The model under review builds one solid part; all positions refer to its coordinate system, in mm. A direction names the side the tool comes from. Coordinates: 2 decimals unless noted, no trailing zeros. Order: outer loops, then holes, each group sorted by start corner. A loop starts at its lowest first (then second) coordinate and runs counter-clockwise, first axis right, second up. Notation, with made-up numbers: (17.25, 17.5) -> (72.25, 17.5) arc R14 cw to (72.25, 31.5) -> close; hole circle Ø11 at (84, 83.5). An arc over 180 degrees is marked (long way). Use one line per item in the form item = value. Start each with the question number.
(1) Mouldability with a two-part tool opening along Z and no side actions: class faces 3 (the flat face through (0, 2, -6)), 4 (the flat face through (-5.3, 5, -4.1)), 5 (the cylindrical face through (1.352, 2.606, 4.292)) as +Z half, -Z half, draft (parallel to the pull), parting line (faces both ways), or undercut.
(2) Take a section at A-A (y = 3.5). State the section outline as (x, z) points, then the cut area to 3 significant figures.
(3) Take a section at C-C (x = 7). State the section outline as (y, z) points, then the cut area to 3 significant figures.
(4) Take a section at D-D (y = 1.45). State the section outline as (x, z) points.
(5) Wall thickness on line 1 along X through (y, z) = (0.95, 0); line 2 along Z through (x, y) = (0, 2.5); line 3 along X through (y, z) = (2.75, 0): over which ranges is each line inside the solid? List them lowest first.
(6) Insertion check: pin 1 Ø4.5 at (x, z) = (-7, 1) entering from +Y. The pin has a flat end and moves straight along its axis. Give the tip position at first contact, or say it passes through.
(7) Take a section at B-B (z = 0.5). State the section outline as (x, y) points.
(8) For faces 1 (the flat face through (-22.5, 2, 0)), 2 (the cylindrical face through (-20.15, 4.01, -0.06)), list the 3-axis set-ups (+Z, -Z, +X, -X, +Y, -Y) from which the entire face can be reached by the end or side of a thin tool; tool diameter is ignored.
```python
from build123d import *

# Parameters (mm, degrees)
SKETCH1_W           = 45
SKETCH1_H           = 12
BOSS_EXTRUDE1_DEPTH = 5
SKETCH2_R           = 2.65
CUT_EXTRUDE1_DEPTH  = 2
SKETCH3_R           = 1.65
CUT_EXTRUDE2_DEPTH  = 12
SKETCH4_R           = 4.5
CUT_EXTRUDE3_DEPTH  = 0.8


with BuildPart() as part:
    # Sketch1 → Boss-Extrude1 (new body)
    with BuildSketch(Plane(origin=(0, 0, 0), x_dir=(1, 0, 0), z_dir=(0, 1, 0))):
        Rectangle(SKETCH1_W, SKETCH1_H)
    extrude(amount=BOSS_EXTRUDE1_DEPTH)

    # Sketch2 → Cut-Extrude1 (cut)
    with BuildSketch(Plane(origin=(0, 5, 0), x_dir=(1, 0, 0), z_dir=(0, 1, 0))):
        with Locations((-17.5, 0)):
            Circle(SKETCH2_R)
        with BuildLine():
            Line((-0.940913384, 4.400532014), (-17.5, 2.65))
            ThreePointArc((-17.5, 2.65), (-15.62616703, 1.87383297), (-14.85, 0))
            ThreePointArc((-14.85, 0), (-15.62616703, -1.87383297), (-17.5, -2.65))
            Line((-17.5, -2.65), (-0.940913384, -4.400532014))
            ThreePointArc((-0.940913384, -4.400532014), (-4.5, 0), (-0.940913384, 4.400532014))
        make_face()
        with BuildLine():
            Line((0, 4.5), (-0.940913384, 4.400532014))
            ThreePointArc((-0.940913384, 4.400532014), (-4.5, 0), (-0.940913384, -4.400532014))
            Line((-0.940913384, -4.400532014), (0, -4.5))
            Line((0, -4.5), (0.940913384, -4.400532014))
            ThreePointArc((0.940913384, -4.400532014), (3.498864832, -2.829831247), (4.5, 0))
            ThreePointArc((4.5, 0), (3.498864832, 2.829831247), (0.940913384, 4.400532014))
            Line((0.940913384, 4.400532014), (0, 4.5))
        make_face()
        with BuildLine():
            Line((17.5, 2.65), (0.940913384, 4.400532014))
            ThreePointArc((0.940913384, 4.400532014), (3.498864832, 2.829831247), (4.5, 0))
            ThreePointArc((4.5, 0), (3.498864832, -2.829831247), (0.940913384, -4.400532014))
            Line((0.940913384, -4.400532014), (17.5, -2.65))
            ThreePointArc((17.5, -2.65), (14.85, 0), (17.5, 2.65))
        make_face()
        with Locations((17.5, 0)):
            Circle(SKETCH2_R)
    extrude(amount=-CUT_EXTRUDE1_DEPTH, mode=Mode.SUBTRACT)

    # Sketch3 → Cut-Extrude2 (cut)
    with BuildSketch(Plane(origin=(0, 3, 0), x_dir=(1, 0, 0), z_dir=(0, 1, 0))):
        with Locations(Location((0, 0, 0), (0, 0, 270))):
            Circle(SKETCH3_R)
    extrude(amount=-CUT_EXTRUDE2_DEPTH, mode=Mode.SUBTRACT)

    # Sketch4 → Cut-Extrude3 (cut)
    with BuildSketch(Plane(origin=(0, 3, 0), x_dir=(1, 0, 0), z_dir=(0, 1, 0))):
        with Locations(Location((0, 0, 0), (0, 0, 270))):
            Circle(SKETCH4_R)
    extrude(amount=-CUT_EXTRUDE3_DEPTH, mode=Mode.SUBTRACT)


solid = part.part
```
Findings:
q1.face_3 = -Z half
q1.face_4 = draft
q1.face_5 = undercut
q2.outline = (-22.5, -6) -> (22.5, -6) -> (22.5, 6) -> (-22.5, 6) -> close; hole (-17.5, -2.65) -> (0, -4.5) -> (17.5, -2.65) arc R2.65 ccw to (17.5, 2.65) -> (0, 4.5) -> (-17.5, 2.65) arc R2.65 ccw to start
q2.area = 268 mm²
q3.outline = (0, -6) -> (5, -6) -> (5, -3.76) -> (3, -3.76) -> (3, 3.76) -> (5, 3.76) -> (5, 6) -> (0, 6) -> close
q3.area = 45.0 mm²
q4.outline = (-22.5, -6) -> (22.5, -6) -> (22.5, 6) -> (-22.5, 6) -> close; hole circle Ø3.3 at (0, 0)
q5.line_1 = -22.5 to -1.65, 1.65 to 22.5
q5.line_2 = -6 to -4.5, 4.5 to 6
q5.line_3 = -22.5 to -4.5, 4.5 to 22.5
q6.pin_1 = 3
q7.outline = (-22.5, 0) -> (-1.57, 0) -> (-1.57, 2.2) -> (-4.47, 2.2) -> (-4.47, 3) -> (-20.1, 3) -> (-20.1, 5) -> (-22.5, 5) -> close; (1.57, 0) -> (22.5, 0) -> (22.5, 5) -> (20.1, 5) -> (20.1, 3) -> (4.47, 3) -> (4.47, 2.2) -> (1.57, 2.2) -> close
q8.face_1 = +Z, -Z, -X, +Y, -Y
q8.face_2 = +Y
